from build123d import *

# Parameters (mm, degrees)
SKETCH1_W                                           = 85
SKETCH1_H                                           = 50.00000000000001
BOSS_EXTRUDE1_DEPTH                                 = 20
CUT_EXTRUDE1_DEPTH                                  = 10
FILLET1_R                                           = 5
FILLET2_R                                           = 10
SKETCH3_R                                           = 12.75
CUT_EXTRUDE2_DEPTH                                  = 10
SKETCH13_R                                          = 3.999999999999999
SKETCH13_R_2                                        = 4.000000000000006
SKETCH13_R_3                                        = 4
CUT_EXTRUDE4_DEPTH                                  = 10
CBORE_FOR_M4_HEX_SOCKET_HEAD_CAP_SCREW2_D           = 4.5
CBORE_FOR_M4_HEX_SOCKET_HEAD_CAP_SCREW2_CBORE_D     = 8
CBORE_FOR_M4_HEX_SOCKET_HEAD_CAP_SCREW2_CBORE_DEPTH = 4.4
FILLET4_R                                           = 5
SKETCH17_R                                          = 14
CUT_EXTRUDE5_DEPTH                                  = 8
SKETCH18_R                                          = 10.000000000000002
CUT_EXTRUDE6_DEPTH                                  = 6
SKETCH19_R                                          = 1.7500000000000038
CUT_EXTRUDE7_DEPTH                                  = 12
FILLET5_R                                           = 1.5
SKETCH20_R                                          = 1.7500000000000004
SKETCH20_R_2                                        = 1.7500000000000002
SKETCH20_R_3                                        = 1.7500000000000038
SKETCH20_R_4                                        = 1.7500000000000036
CUT_EXTRUDE8_DEPTH                                  = 7


with BuildPart() as part:
    # Sketch1 → Boss-Extrude1 (new body)
    with BuildSketch(Plane(origin=(0, 0, 0), x_dir=(1, 0, 0), z_dir=(0, 1, 0))):
        Rectangle(SKETCH1_W, SKETCH1_H)
    extrude(amount=BOSS_EXTRUDE1_DEPTH)

    # Sketch2 → Cut-Extrude1 (cut)
    with BuildSketch(Plane(origin=(0, 20, 0), x_dir=(1, 0, 0), z_dir=(0, 1, 0))):
        with BuildLine():
            ThreePointArc((-5.41666666666668, 9.67348897186992), (-37.500000000000014, 2.14e-15), (-5.41666666666668, -9.67348897186992))
            ThreePointArc((-5.41666666666668, -9.67348897186992), (39.499999999999986, 0), (-5.41666666666668, 9.67348897186992))
        make_face()
    extrude(amount=-CUT_EXTRUDE1_DEPTH, mode=Mode.SUBTRACT)

    # Fillet1
    fillet1_edges = [part.edges().sort_by_distance(p)[0] for p in [
        (42.5, 10, 25),
        (-42.5, 10, 25),
        (-42.5, 10, -25),
        (42.5, 10, -25),
    ]]
    fillet(fillet1_edges, radius=FILLET1_R)

    # Fillet2
    fillet2_edges = [part.edges().sort_by_distance(p)[0] for p in [
        (-5.4166666666666785, 15, -9.673488971869928),
        (-5.416666666666677, 15, 9.673488971869919),
    ]]
    fillet(fillet2_edges, radius=FILLET2_R)

    # Sketch3 → Cut-Extrude2 (cut)
    with BuildSketch(Plane(origin=(0, 10, 0), x_dir=(1, 0, 0), z_dir=(0, 1, 0))):
        with Locations(Location((-20.00000000000001, 0, 0), (0, 0, 270))):
            Circle(SKETCH3_R)
    extrude(amount=-CUT_EXTRUDE2_DEPTH, mode=Mode.SUBTRACT)

    # Sketch13 → Cut-Extrude4 (cut)
    with BuildSketch(Plane(origin=(0, 10, 0), x_dir=(1, 0, 0), z_dir=(0, 1, 0))):
        with Locations((-20.00000000000001, 17.500000000000004)):
            Circle(SKETCH13_R)
        with Locations((-37.50000000000002, 0)):
            Circle(SKETCH13_R_2)
        with Locations((-20.00000000000001, -17.500000000000004)):
            Circle(SKETCH13_R)
        with Locations((-2.5000000000000058, 0)):
            Circle(SKETCH13_R_3)
    extrude(amount=CUT_EXTRUDE4_DEPTH, mode=Mode.SUBTRACT)

    # CBORE for M4 Hex Socket Head Cap Screw2 (through all)
    with Locations(Plane(origin=(0, 10, 0), x_dir=(1, 0, 0), z_dir=(0, 1, 0))):
        with Locations((-20, 17.5), (-37.5, 0), (-20, -17.5), (-2.5, 0)):
            CounterBoreHole(CBORE_FOR_M4_HEX_SOCKET_HEAD_CAP_SCREW2_D / 2, CBORE_FOR_M4_HEX_SOCKET_HEAD_CAP_SCREW2_CBORE_D / 2, CBORE_FOR_M4_HEX_SOCKET_HEAD_CAP_SCREW2_CBORE_DEPTH)

    # Fillet4
    # the kernel refuses this fillet: 5 mm, written as the material it takes off along each edge
    with BuildSketch(Plane(origin=(-23.973791691591714, 10, -17.042857142857144), x_dir=(-0.954076861711662, 0, 0.2995619167157709), z_dir=(0, 1, 0))) as fillet4_piece_1:
        with BuildLine():
            CenterArc((3.0036302761545866, -4.985883518062786), FILLET4_R, 94.30643699703337, 46.066169411844314)
            ThreePointArc((-0.847411708769257, -1.796921989546989), (-0.3103690050239528, -0.9519095995220337), (0, 0))
            ThreePointArc((0, 0), (1.3140882458176382, -0.04940768678026136), (2.6281764916352697, 5e-17))
        make_face()
    extrude(amount=16.570441229088175, mode=Mode.SUBTRACT)
    with BuildSketch(Plane(origin=(-16.026208308408307, 10, -17.042857142857148), x_dir=(0.9540768617116616, 0, 0.2995619167157718), z_dir=(0, 1, 0))) as fillet4_piece_2:
        with BuildLine():
            CenterArc((3.0036302761545857, 4.985883518062786), FILLET4_R, 219.62739359112237, 46.06616941184433)
            ThreePointArc((-0.8474117087692576, 1.7969219895469846), (-0.31036900502395265, 0.95190959952203), (0, 0))
            ThreePointArc((0, 0), (1.3140882458176364, 0.04940768678026209), (2.628176491635274, 4e-17))
        make_face()
    extrude(amount=16.570441229088186, mode=Mode.SUBTRACT)
    with BuildSketch(Plane(origin=(-37.04285714285715, 10, 3.973791691591705), x_dir=(0.29956191671576937, 0, 0.9540768617116623), z_dir=(0, 1, 0))) as fillet4_piece_3:
        with BuildLine():
            CenterArc((3.0036302761546088, -4.985883518062785), FILLET4_R, 94.30643699703347, 46.06616941184433)
            ThreePointArc((-0.8474117087692441, -1.7969219895469968), (-0.3103690050239449, -0.9519095995220361), (0, 0))
            ThreePointArc((0, 0), (1.3140882458176406, -0.04940768678026007), (2.628176491635283, 2e-17))
        make_face()
    extrude(amount=16.57044122908821, mode=Mode.SUBTRACT)
    with BuildSketch(Plane(origin=(-37.04285714285716, 10, -3.9737916915917033), x_dir=(-0.9907079173697112, 0, 0.13600670005911286), z_dir=(0, 1, 0))) as fillet4_piece_4:
        with BuildLine():
            CenterArc((3.2284113635675427, -4.843365499227848), FILLET4_R, 104.37926436272748, 46.066169411844285)
            ThreePointArc((-1.1210203197438697, -2.377104354862376), (-0.51582243521462, -1.2096264930292784), (0, 0))
            ThreePointArc((0, 0), (0.9933573426361664, -0.12530760061772306), (1.986714685272327, 0))
        make_face()
    extrude(amount=16.570441229088196, mode=Mode.SUBTRACT)
    with BuildSketch(Plane(origin=(-16.026208308408307, 10, 17.042857142857144), x_dir=(0.9540768617116622, 0, -0.29956191671577), z_dir=(0, 1, 0))) as fillet4_piece_5:
        with BuildLine():
            CenterArc((3.003630276154599, -4.985883518062785), FILLET4_R, 94.30643699703343, 46.06616941184434)
            ThreePointArc((-0.8474117087692495, -1.7969219895469952), (-0.31036900502395187, -0.9519095995220339), (0, 0))
            ThreePointArc((0, 0), (1.314088245817627, -0.04940768678026029), (2.6281764916352777, 1e-17))
        make_face()
    extrude(amount=16.570441229088196, mode=Mode.SUBTRACT)
    with BuildSketch(Plane(origin=(-23.97379169159171, 10, 17.042857142857144), x_dir=(0.1360067000591155, 0, 0.9907079173697108), z_dir=(0, 1, 0))) as fillet4_piece_6:
        with BuildLine():
            CenterArc((3.2284113635675378, -4.843365499227849), FILLET4_R, 104.37926436272741, 46.06616941184424)
            ThreePointArc((-1.1210203197438684, -2.37710435486237), (-0.5158224352146136, -1.2096264930292846), (0, 0))
            ThreePointArc((0, 0), (0.9933573426361628, -0.12530760061772173), (1.9867146852723276, -3e-17))
        make_face()
    extrude(amount=16.570441229088182, mode=Mode.SUBTRACT)

    # Sketch17 → Cut-Extrude5 (cut)
    with BuildSketch(Plane(origin=(0, 10, 0), x_dir=(1, 0, 0), z_dir=(0, 1, 0))):
        with Locations(Location((15.999999999999986, 0, 0), (0, 0, 270))):
            Circle(SKETCH17_R)
    extrude(amount=-CUT_EXTRUDE5_DEPTH, mode=Mode.SUBTRACT)

    # Sketch18 → Cut-Extrude6 (cut)
    with BuildSketch(Plane(origin=(0, 2, 0), x_dir=(1, 0, 0), z_dir=(0, 1, 0))):
        with Locations(Location((15.999999999999986, 0, 0), (0, 0, 270))):
            Circle(SKETCH18_R)
    extrude(amount=-CUT_EXTRUDE6_DEPTH, mode=Mode.SUBTRACT)

    # Sketch19 → Cut-Extrude7 (cut)
    with BuildSketch(Plane(origin=(0, 20, 0), x_dir=(1, 0, 0), z_dir=(0, 1, 0))):
        with Locations(Location((-37.49770482679156, 19.999999999999996, 0), (0, 0, 270))):
            Circle(SKETCH19_R)
        with Locations(Location((37.50229517320846, 20, 0), (0, 0, 270))):
            Circle(SKETCH19_R)
        with Locations(Location((37.50229517320845, -20, 0), (0, 0, 270))):
            Circle(SKETCH19_R)
        with Locations(Location((-37.49770482679156, -20, 0), (0, 0, 270))):
            Circle(SKETCH19_R)
    extrude(amount=-CUT_EXTRUDE7_DEPTH, mode=Mode.SUBTRACT)

    # Fillet5
    fillet5_edges = [part.edges().sort_by_distance(p)[0] for p in [
        (42.5, 0, 0),
        (0, 0, 25),
        (-42.5, 0, 0),
        (0, 0, -25),
        (-41.03553390593274, 0, -23.535533905932738),
        (41.03553390593274, 0, -23.535533905932738),
        (-41.03553390593274, 0, 23.535533905932738),
        (41.03553390593274, 0, 23.535533905932738),
    ]]
    fillet(fillet5_edges, radius=FILLET5_R)

    # Sketch20 → Cut-Extrude8 (cut)
    with BuildSketch(Plane.XY.offset(25)):
        with Locations((-30, 15.75)):
            Circle(SKETCH20_R)
        with Locations((-30, 5.750000000000002)):
            Circle(SKETCH20_R_2)
        with Locations((30, 15.75)):
            Circle(SKETCH20_R_3)
        with Locations((30, 5.750000000000002)):
            Circle(SKETCH20_R_4)
    cut_extrude8 = extrude(amount=-CUT_EXTRUDE8_DEPTH, mode=Mode.SUBTRACT)

    # Mirror1: Cut-Extrude8 across plane
    add(cut_extrude8.mirror(Plane.XY), mode=Mode.SUBTRACT)


solid = part.part
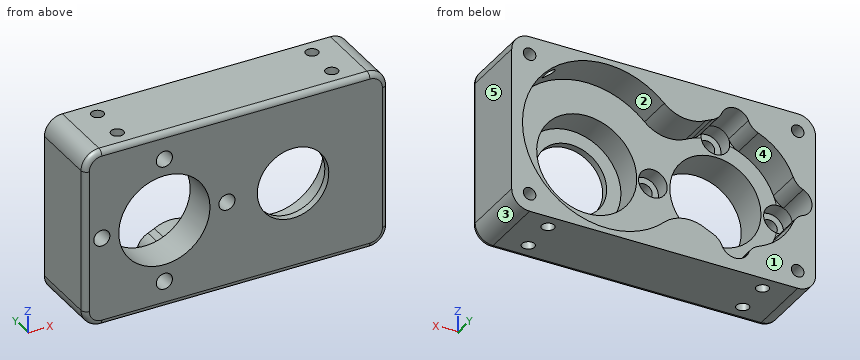
Input: part model. Units: mm. Frame: model coordinates. Face numbers are marked on the shaded views. A direction names the side the tool comes from. Coordinates: 2 decimals unless noted, no trailing zeros. Loops run counter-clockwise (first coordinate to the right, second up) from the corner with the lowest first, then second, coordinate; pieces in that order, holes last.
(1) Section C-C on z = 0. Count the separate pieces of the cut face and the enclosed holes in it, then the cut area to 3 significant figures.
(2) Section A-A on x = -20. Return the cut outline in (y, z), then the cut area to 3 significant figures.
(3) First-contact query: pin 1 Ø3 at (x, y) = (30, 5.75) entering from -Z; pin 2 Ø4 at (x, z) = (27, 14.5) entering from +Y; pin 3 Ø6.5 at (x, z) = (-20, -17.5) entering from +Y. Flat tips, straight axial feed; report the tip coordinate or a pass-through.
(4) Set-up query: the marked faces 4 and 5. Return all of +Z, -Z, +X, -X, +Y, -Y with unobstructed straight access to the full face (end or side cutting, diameter ignored); none if empty.
(5) Section B-B on x = 16. Return the cut outline in (y, z), then the cut area to 3 significant figures.
(6) Material intervals for probe 1 along Y at (x, z) = (-30, 23.25); probe 2 along Z at (x, y) = (-13.5, 19); probe 3 along X at (y, z) = (9, -19), sorted ascending.
(7) Pull-direction query (X, two-part tool) for the marked faces 1, 2 and 3; classes: released by +X, released by -X, zero draft, split by the parting line, or undercut.
Data:
1. separate pieces: 5
1. enclosed holes: 0
1. area: 249 mm2
2. outline: (0, -23.5) arc R1.5 ccw to (1.5, -25) - (20, -25) - (20, -21.5) - (5.6, -21.5) - (5.6, -19.75) - (0, -19.75) - close; (0, -15.25) - (5.6, -15.25) - (5.6, -13.5) - (10, -13.5) - (10, -12.75) - (0, -12.75) - close; (0, 12.75) - (10, 12.75) - (10, 13.5) - (5.6, 13.5) - (5.6, 15.25) - (0, 15.25) - close; (0, 19.75) - (5.6, 19.75) - (5.6, 21.5) - (20, 21.5) - (20, 25) - (1.5, 25) arc R1.5 ccw to (0, 23.5) - close
2. area: 193 mm2
3. pin 1: stops at z = -18
3. pin 2: stops at y = 10
3. pin 3: stops at y = 5.6
4. face 4: +Y
4. face 5: +Z, -Z, +X, +Y, -Y
5. outline: (0, -23.5) arc R1.5 ccw to (1.5, -25) - (20, -25) - (20, -23.5) - (10, -23.5) - (10, -14) - (2, -14) - (2, -10) - (0, -10) - close; (0, 10) - (2, 10) - (2, 14) - (10, 14) - (10, 23.5) - (20, 23.5) - (20, 25) - (1.5, 25) arc R1.5 ccw to (0, 23.5) - close
5. area: 265 mm2
6. probe 1: y = 0 to 4, 7.5 to 14, 17.5 to 20
6. probe 2: z = -25 to -16.25, 16.25 to 25
6. probe 3: x = -42.5 to -38.93, -36.06 to -23.71, -16.29 to 36.07, 38.94 to 42.5
7. face 1: zero draft
7. face 2: undercut
7. face 3: released by +X
